```python
from build123d import *

# Parameters (mm, degrees)
F0_R     = 28.575
F1_DEPTH = 64
F0_R_2   = 11.1
F2_DEPTH = 44
F3_W     = 114
F3_H     = 50
F4_DEPTH = 22
F5_SIZE  = 12
F7_DEPTH = 10
F8_SIZE  = 12


# Not quite as in the source:
# - after a boolean that leaves OpenCascade's solid faulty, fix() repairs it


with BuildPart() as f1:
    # F0 (on Front) → F1 (new body)
    with BuildSketch(Plane.XZ):
        with BuildLine():
            ThreePointArc((35.1425667816, -41), (49.0596504584, -22.5643678594), (54, 0))
            ThreePointArc((54, 0), (49.0596504584, 22.5643678594), (35.1425667816, 41))
            ThreePointArc((35.1425667816, 41), (-54, 0), (35.1425667816, -41))
        make_face()
        Circle(F0_R, mode=Mode.SUBTRACT)
    extrude(amount=F1_DEPTH)

    # F0 (on Front) → F2 (join)
    with BuildSketch(Plane.XZ):
        with BuildLine():
            ThreePointArc((35.1425667816, 41), (49.0596504584, 22.5643678594), (54, 0))
            ThreePointArc((54, 0), (49.0596504584, -22.5643678594), (35.1425667816, -41))
            Line((35.1425667816, -41), (174, -41))
            Line((174, -41), (174, 41))
            Line((174, 41), (35.1425667816, 41))
        make_face()
        with Locations((89, 0)):
            Circle(F0_R_2, mode=Mode.SUBTRACT)
        with Locations((139, 0)):
            Circle(F0_R_2, mode=Mode.SUBTRACT)
    extrude(amount=F2_DEPTH)

    # F3 (on face) → F4 (cut)
    with BuildSketch(Plane.XZ.offset(44)):
        with Locations((117, 0)):
            Rectangle(F3_W, F3_H)
    extrude(amount=-F4_DEPTH, mode=Mode.SUBTRACT)

    # F5
    f5_edges = [f1.edges().sort_by_distance(p)[0] for p in [
        (174, -44, -33),
    ]]
    chamfer(f5_edges, length=F5_SIZE)

    # F6 (on face) → F7 (join)
    with BuildSketch(Plane.XZ.offset(64)):
        with BuildLine():
            Line((-23.6755279772, 16), (-51.5751878329, 16))
            ThreePointArc((-51.5751878329, 16), (-54, 0), (-51.5751878329, -16))
            Line((-51.5751878329, -16), (-23.6755279772, -16))
            ThreePointArc((-23.6755279772, -16), (-28.575, 0), (-23.6755279772, 16))
        make_face()
        with BuildLine():
            Line((51.5751878329, 16), (23.6755279772, 16))
            ThreePointArc((23.6755279772, 16), (28.575, 0), (23.6755279772, -16))
            Line((23.6755279772, -16), (51.5751878329, -16))
            ThreePointArc((51.5751878329, -16), (54, 0), (51.5751878329, 16))
        make_face()
    extrude(amount=F7_DEPTH)

    add(f1.part.fix(), mode=Mode.REPLACE)

    # F8
    f8_edges = [f1.edges().sort_by_distance(p)[0] for p in [
        (174, -44, 33),
    ]]
    chamfer(f8_edges, length=F8_SIZE)


solid = f1.part
```
The model under review builds one solid part; all positions refer to its coordinate system, in mm. A direction names the side the tool comes from. Round coordinates to 2 decimals unless told otherwise and drop trailing zeros. Loops run counter-clockwise (first coordinate to the right, second up) from the corner with the lowest first, then second, coordinate; pieces in that order, holes last. Notation, with made-up numbers: M 85,45 L 97,45 A11 ccw 97,58 Z; hole C 5.25,48 d9. An arc over 180 degrees is marked long. Write item = value, one per line.
Item 1: Take a section at C-C on y = -19. Write out the cut boundary in (x, z) (3 decimals), then the cut area to 3 significant figures.
Return value:
outline = M 35.143,-41 L 174,-41 L 174,41 L 35.143,41 A54 ccw long Z; hole C 0,0 d57.15; hole C 89,0 d22.2; hole C 139,0 d22.2
area = 16,100 mm2
Item 2: Take a section at B-B on x = 0. Write out the cut boundary in (y, z) (3 decimals), then the cut area to 3 significant figures.
Return value:
outline = M -64,-54 L 0,-54 L 0,-28.575 L -64,-28.575 Z; M -64,28.575 L 0,28.575 L 0,54 L -64,54 Z
area = 3,250 mm2
Item 3: Take a section at D-D on x = 159. Write out the cut boundary in (y, z), then the cut area to 3 significant figures.
Return value:
outline = M -44,-41 L 0,-41 L 0,41 L -44,41 L -44,25 L -22,25 L -22,-25 L -44,-25 Z
area = 2,510 mm2
Item 4: For line 1 (X direction, y = -10, z = 0) (3 decimals); line 2 (X direction, y = -61, z = -16); line 3 (Z direction, x = 89, y = -17.25), list the stretches that pass through material, from the lowest coordinate up. Write a range as [from, to].
Return value:
line_1 = [-54, -28.575], [28.575, 77.9], [100.1, 127.9], [150.1, 174]
line_2 = [-51.58, -23.68], [23.68, 51.58]
line_3 = [-41, -11.1], [11.1, 41]
Item 5: The part is to be moulded in two halves that separate along X. For faces 1 (the flat face through (174, -12, -1)), 2 (the cylindrical face through (127.91, -10.85, 0.49)), 3 (the cylindrical face through (-52.836, -36.482, 11.152)), 4 (the flat face through (-39, -74, 0)), say which applies: released by +X, released by -X, zero draft, split by the parting line, or undercut.
Return value:
face_1 = released by +X
face_2 = undercut
face_3 = split by the parting line
face_4 = zero draft
Item 6: Insertion check: P1, Ø5, axis at y = -63, z = 34.5, coming from the -X side; P2, Ø3, axis at y = -66, z = -5.5, coming from the -X side; P3, Ø5, axis at x = -42, y = -68, coming from the +Z side; P4, Ø17.5, axis at y = -28.5, z = -8, coming from the +X side. Each pin has a flat end and moves straight along its axis. Give the tip position at first contact, or say it passes through.
Return value:
P1 = -43.5
P2 = -53.85
P3 = 16
P4 = 174
Item 7: Machinability: for faces 5 (the flat face through (116, -33, 25)), 6 (the flat face through (-37, -69, 16)), 7 (the flat face through (106, -22, 41)), 8 (the flat face through (104, -22, -41)), which of the approach directions +Z, -Z, +X, -X, +Y, -Y give a long, thin tool a straight path to every point of the face, cutting with its end or side? Answer none if there is none.
Return value:
face_5 = +X, -Y
face_6 = +Z, +X, -X, -Y
face_7 = +Z, +X, +Y, -Y
face_8 = -Z, +X, +Y, -Y
Item 8: Take a section at A-A on z = 0. Write out the cut boundary in (x, y) (3 decimals).
Return value:
outline = M -54,-74 L -28.575,-74 L -28.575,0 L -54,0 Z; M 28.575,-74 L 54,-74 L 54,-44 L 60,-44 L 60,-22 L 77.9,-22 L 77.9,0 L 28.575,0 Z; M 100.1,-22 L 127.9,-22 L 127.9,0 L 100.1,0 Z; M 150.1,-22 L 174,-22 L 174,0 L 150.1,0 Z
